For this review, use the dimensioned drawing (mm, ordinates from the lowest corner) and the shaded views. Coordinates: 2 decimals unless noted, no trailing zeros. Order: outer loops, then holes, each group sorted by start corner. A loop starts at its lowest first (then second) coordinate and runs counter-clockwise, first axis right, second up. Notation, with made-up numbers: M 74.5,-4.75 L 115.5,-4.75 A19 cw 115.5,15.25 Z; hole C 52,31 d1. An arc over 180 degrees is marked long. Answer as CSV lines item,"result". Start each with the question number.
Q1. Consider section A-A on z = 15. Write out the cut boundary in (x, y).
Q2. For P1, Ø2, axis at y = 19, z = 11, coming from the +X side, flat-tipped, find the tip position at first contact; note if it passes through.
Q3. Consider section C-C on x = 16.5. Write out the cut boundary in (y, z).
Q4. The part is to be moulded in two halves that separate along Z. For the marked faces 1, 2, 3 and 4, say which applies: +Z half, -Z half, draft (parallel to the pull), parting line (faces both ways), or undercut.
Q5. Wall thickness on L1, parallel to Y at x = 14, z = 18; L2, parallel to Y at x = 13, z = 16.75; L3, parallel to Z at x = 6, y = 12.25: over which ranges is each line inside the solid? List them lowest first. Write a range as [from, to].
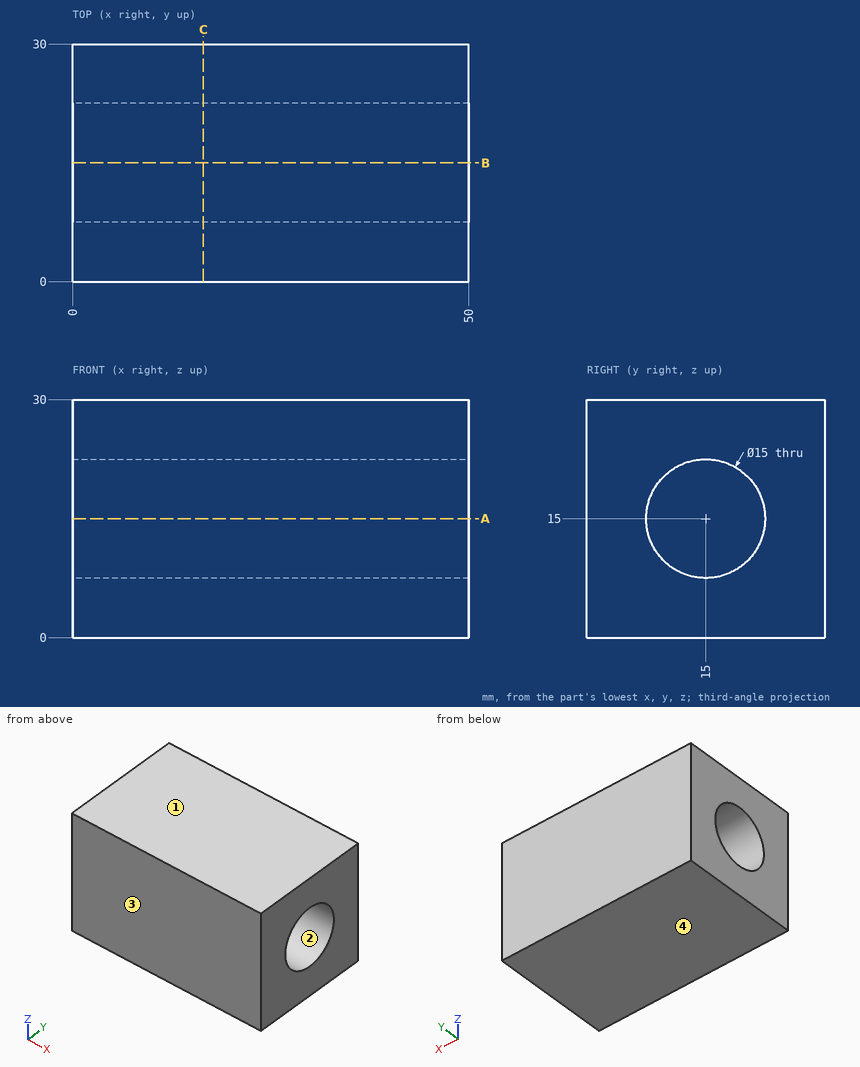
Evaluation:
1,outline,"M 0,0 L 50,0 L 50,7.5 L 0,7.5 Z; M 0,22.5 L 50,22.5 L 50,30 L 0,30 Z"
2,P1,"passes through"
3,outline,"M 0,0 L 30,0 L 30,30 L 0,30 Z; hole C 15,15 d15"
4,face 1,"+Z half"
4,face 2,"undercut"
4,face 3,"draft"
4,face 4,"-Z half"
5,L1,"y = [0, 8.13], [21.87, 30]"
5,L2,"y = [0, 7.71], [22.29, 30]"
5,L3,"z = [0, 8.02], [21.98, 30]"
